Model file for the job. Use its own axes, mm. A direction names the side the tool comes from. Round coordinates to 2 decimals unless told otherwise and drop trailing zeros. Order: outer loops, then holes, each group sorted by start corner. A loop starts at its lowest first (then second) coordinate and runs counter-clockwise, first axis right, second up. Notation, with made-up numbers: (44, -37.75) - (95, -37.75) arc R14 cw to (95, -17.75) - close; hole circle Ø4 at (-6.5, -16). An arc over 180 degrees is marked (long way). Use one line per item in the form item = value.
from build123d import *

# Parameters (mm, degrees)
CUT_EXTRUDE1_DEPTH = 5.08
CIRPATTERN1_COUNT  = 3


# Read off the part's stored shape, not the designer's step: Revolve1
with BuildPart() as part:
    # Revolve1 outline → Revolve1 (revolve)
    with BuildSketch(Plane.YX):
        Polygon((20.701, 7.62), (19.430746, 7.62), (19.430746, 293.37), (18.160746, 293.37), (18.160746, 5.08), (18.161, 5.08), (18.161, 0), (20.701, 0), align=None)
    revolve(axis=Axis((0, 0, 0), (1, 0, 0)))

    # Sketch2 → Cut-Extrude1 (cut)
    with BuildSketch(Plane(origin=(0, 19.430746, 0), x_dir=(1, 0, 0), z_dir=(0, 1, 0))):
        with BuildLine():
            Line((20.6375, 3.175), (20.6375, -3.175))
            ThreePointArc((20.6375, -3.175), (19.05, -4.7625), (17.4625, -3.175))
            Line((17.4625, -3.175), (17.4625, 3.175))
            ThreePointArc((17.4625, 3.175), (19.05, 4.7625), (20.6375, 3.175))
        make_face()
    cut_extrude1 = extrude(amount=-CUT_EXTRUDE1_DEPTH, mode=Mode.SUBTRACT)

    # CirPattern1: Cut-Extrude1 ×3 about axis
    cirpattern1_axis = Axis((0, 0, 0), (-1, 0, 0))
    for i in range(1, CIRPATTERN1_COUNT):
        add(cut_extrude1.rotate(cirpattern1_axis, i * 360 / CIRPATTERN1_COUNT), mode=Mode.SUBTRACT)


solid = part.part
(1) Tool access for faces 1 (the face through (2.504, 9.763, 15.313)), 2 (the face through (152.495, -19.412, 0.854)): list every direction of +Z, -Z, +X, -X, +Y, -Y with a clear straight run to the whole face (end or side of a thin tool).
Report:
face_1 = +X, -X
face_2 = +X
(2) Pull direction Z, two halves, no side cores. Call faces 3 (the face through (3.863, -16.428, -12.596)), 4 (the face through (0, -1.4, -18.3)), 5 (the face through (147.2, 8.4, -16.1)): released by +Z, released by -Z, zero draft, split by the parting line, or undercut.
Report:
face_3 = split by the parting line
face_4 = zero draft
face_5 = undercut
(3) Slice it at A-A on z = 0. Count the separate pieces of the cut face and the enclosed holes in it, then the cut area to 3 significant figures.
Report:
separate_pieces = 3
enclosed_holes = 0
area = 760 mm2
(4) Probe probe 1 along Z at (x, y) = (1.2, 0); probe 2 along Y at (x, z) = (237, 1) (3 decimals); probe 3 along Z at (x, y) = (169, 0). List the from-to ranges inside material, lowest first. Write a range as [from, to].
Report:
probe_1 = [-20.7, -18.16], [18.16, 20.7]
probe_2 = [-19.405, -18.133], [18.133, 19.405]
probe_3 = [-19.43, -18.16], [18.16, 19.43]
(5) Slice it at C-C on x = 57. Give the cut face in (y, z).
Report:
outline = circle Ø38.86 at (0, 0); hole circle Ø36.32 at (0, 0)
(6) Pin check, flat tips, straight feed: pin 1 (1.5 mm diameter, centred on x = 71, y = 1.5, fed in from -Z); pin 2 (4 mm diameter, centred on x = 203, y = 12.5, fed in from +Z); pin 3 (8 mm diameter, centred on x = 158.5, z = -13.5, fed in from -Y). Stop position of each tip, or through.
Report:
pin_1 = -19.42
pin_2 = 16.35
pin_3 = -16.95
